The listing builds one solid part. Answer for the finished solid, in the listing's coordinates (mm). A direction names the side the tool comes from. Coordinates: 2 decimals unless noted, no trailing zeros. Write each loop counter-clockwise with the first axis right and the second up, starting at its lowest first coordinate (ties: lowest second). Pieces come first, ordered by that corner, then holes.
from build123d import *

# Parameters (mm, degrees)
BOSS_EXTRUDE1_DEPTH = 1.5875
SKETCH3_W           = 208.645691316
SKETCH3_H           = 383.026987577
CUT_EXTRUDE1_DEPTH  = 121.20569203
CUT_EXTRUDE2_DEPTH  = 4.175


with BuildPart() as part:
    # Sketch2 → Boss-Extrude1 (new body, symmetric)
    with BuildSketch(Plane.XY):
        with BuildLine():
            ThreePointArc((-120.098895727, 19.05), (0.406748907, 139.2017743), (120.203613722, 18.343301545))
            ThreePointArc((120.203613722, 18.343301545), (101.067699546, -47.629728931), (50.138751442, -93.726))
            ThreePointArc((50.138751442, -93.726), (0.040174098, -101.514794876), (-50.058403246, -93.726))
            ThreePointArc((-50.058403246, -93.726), (-101.163912713, -47.327889321), (-120.098895727, 19.05))
        make_face()
        with BuildLine():
            ThreePointArc((-104.858895727, 19.05), (0.361930242, 123.961840203), (104.963877332, 18.432938489))
            ThreePointArc((104.963877332, 18.432938489), (88.446745877, -39.065849025), (44.40486057, -79.553359885))
            ThreePointArc((44.40486057, -79.553359885), (0.040463589, -86.274794876), (-44.323959374, -79.553531384))
            ThreePointArc((-44.323959374, -79.553531384), (-88.517658334, -38.801393502), (-104.858895727, 19.05))
        make_face(mode=Mode.SUBTRACT)
    extrude(amount=BOSS_EXTRUDE1_DEPTH, both=True)

    # Sketch3 → Cut-Extrude1 (cut, through all)
    with BuildSketch(Plane(origin=(0, 0, 0), x_dir=(0, 0, -1), z_dir=(1, 0, 0))):
        with Locations((4.266053154, 20.866300598)):
            Rectangle(SKETCH3_W, SKETCH3_H)
    extrude(amount=CUT_EXTRUDE1_DEPTH, mode=Mode.SUBTRACT)

    # Sketch4 → Cut-Extrude2 (cut, through all)
    with BuildSketch(Plane.XY.offset(1.5875)):
        with BuildLine():
            Line((-95.442778735, 76.146002016), (-103.1094988, 80.645376586))
            ThreePointArc((-103.1094988, 80.645376586), (-103.96522962, 79.188995674), (-104.80040165, 77.720728574))
            Line((-104.80040165, 77.720728574), (-97.152639859, 73.232480062))
            Line((-97.152639859, 73.232480062), (-95.442778735, 76.146002016))
        make_face()
        with BuildLine():
            Line((-3.3782, 139.153279965), (-3.3782, 130.312293878))
            Line((-3.3782, 130.312293878), (0, 130.312293878))
            Line((0, 130.312293878), (0, 139.202282013))
            ThreePointArc((0, 139.202282013), (-1.689272244, 139.189655502), (-3.3782, 139.153279965))
        make_face()
        with BuildLine():
            Line((-97.044954451, -36.819436689), (-104.679734985, -41.300066711))
            ThreePointArc((-104.679734985, -41.300066711), (-103.859441192, -42.776931517), (-103.019390964, -44.242648808))
            Line((-103.019390964, -44.242648808), (-95.335093375, -39.732958671))
            Line((-95.335093375, -39.732958671), (-97.044954451, -36.819436689))
        make_face()
        with BuildLine():
            Line((-3.302, -92.624794876), (-3.302, -101.48094955))
            ThreePointArc((-3.302, -101.48094955), (-1.651084663, -101.506132106), (0, -101.514794876))
            Line((0, -101.514794876), (0, -92.624794876))
            Line((0, -92.624794876), (-3.302, -92.624794876))
        make_face()
    extrude(amount=-CUT_EXTRUDE2_DEPTH, mode=Mode.SUBTRACT)


solid = part.part
1. Section C-C on y = -5 is taken. Give the vertices of the cut face in (x, z).
Results found:
outline: (-117.78, -1.59) - (-102.21, -1.59) - (-102.21, 1.59) - (-117.78, 1.59) - close
2. Section A-A on x = -9 is taken. Give the vertices of the cut face in (y, z), then the cut area to 3 significant figures.
Results found:
outline: (-101.27, -1.59) - (-86, -1.59) - (-86, 1.59) - (-101.27, 1.59) - close; (123.57, -1.59) - (138.86, -1.59) - (138.86, 1.59) - (123.57, 1.59) - close
area: 97.0 mm2
3. Section D-D on x = -81 is taken. Give the vertices of the cut face in (y, z).
Results found:
outline: (-72.11, -1.59) - (-49.56, -1.59) - (-49.56, 1.59) - (-72.11, 1.59) - close; (85.66, -1.59) - (107.75, -1.59) - (107.75, 1.59) - (85.66, 1.59) - close
4. Flat-ended cylindrical pins translate along their axes: P1, Ø1.6, axis at y = -99, z = 0.5, coming from the +X side; P2, Ø1, axis at x = -26, z = -1, coming from the -Y side. Find the tip coordinate at first contact, or state that the pin passes through.
Results found:
P1: stops at x = -3.3
P2: stops at y = -99.53
5. Find the intervals of material crossed by L1, parallel to Y at x = -72, z = 0.75; L2, parallel to Y at x = -76, z = 0.6; L3, parallel to X at y = -9.5, z = 0, in increasing order.
Results found:
L1: y = -79.89 to -59.61, 95.31 to 115.2
L2: y = -76.61 to -55.44, 91.32 to 112.07
L3: x = -116.82 to -101.11
6. For a pull along X with two mould halves and no side action, classify faces 4 (the flat face through (-101.03, 75.51, 0.02)), 5 (the flat face through (-104, 2, -1.588)), 6 (the flat face through (-99.2, -42, 0)), 7 (the cylindrical face through (-61.471, 122.255, 0.022)) as pulls with the +X half, pulls with the -X half, needs draft (parallel to the pull), parting line crosses it, or undercut.
Results found:
face 4: undercut
face 5: needs draft
face 6: undercut
face 7: pulls with the -X half
7. A tool of negligible diameter and unlimited length cuts with its end or side. For faces 1 (the flat face through (-104, 2, 1.588)), 2 (the flat face through (-100.81, -39.03, 0.02)), 3 (the cylindrical face through (-22.1, -84.63, 0.02)), from which of +Z, -Z, +X, -X, +Y, -Y can it reach the whole face along a straight path? Write none if from no direction.
Results found:
face 1: +Z, +X, -X, +Y, -Y
face 2: +Z, -Z
face 3: +Z, -Z, +X
8. Section B-B on z = -1 is taken. Give the vertices of the cut face in (x, y).
Results found:
outline: (-120.1, 19.05) arc R125.81 ccw to (-104.68, -41.3) - (-97.04, -36.82) - (-95.34, -39.73) - (-103.02, -44.24) arc R125.81 ccw to (-50.06, -93.73) arc R165.01 ccw to (-3.3, -101.48) - (-3.3, -92.62) - (0, -92.62) - (0, -86.27) arc R149.77 cw to (-44.32, -79.55) arc R110.57 cw to (-104.86, 19.05) arc R104.91 cw to (0, 123.96) - (0, 130.31) - (-3.38, 130.31) - (-3.38, 139.15) arc R120.15 ccw to (-103.11, 80.65) - (-95.44, 76.15) - (-97.15, 73.23) - (-104.8, 77.72) arc R120.15 ccw to start
